Input: part model. Units: mm. Frame: model coordinates. Face numbers are marked on the shaded views. A direction names the side the tool comes from. Round coordinates to 2 decimals unless told otherwise and drop trailing zeros. Order: outer loops, then holes, each group sorted by start corner. A loop starts at its lowest first (then second) coordinate and runs counter-clockwise, first axis right, second up. Notation, with made-up numbers: (72.5, 29.5) - (103.5, 29.5) arc R18 ccw to (103.5, 37.5) - close; hole circle Ø11 at (87.25, 61.5). An arc over 180 degrees is marked (long way). One line per item, written item: value. Start each with the question number.
from build123d import *
from build123d.topology import SkipClean

# Parameters (mm, degrees)
BOSS_EXTRUDE1_DEPTH = 3.3
SKETCH2_R           = 8.19
BOSS_EXTRUDE2_DEPTH = 2.6
BOSS_EXTRUDE3_DEPTH = 1.2
BOSS_EXTRUDE4_DEPTH = 1
SKETCH7_R           = 5.575
BOSS_EXTRUDE5_DEPTH = 1
BOSS_EXTRUDE6_DEPTH = 1.6
BOSS_EXTRUDE7_DEPTH = 3.3
SKETCH9_R           = 3.43
BOSS_EXTRUDE8_DEPTH = 6.5
BOSS_EXTRUDE9_START = 0.65
BOSS_EXTRUDE9_DEPTH = 0.65


with BuildPart() as part:
    # Sketch1 → Boss-Extrude1 (new body)
    with BuildSketch(Plane(origin=(0, 0, 0), x_dir=(1, 0, 0), z_dir=(0, 1, 0))):
        with BuildLine():
            Line((8.141120253, -0.893454545), (6.690358093, -0.893454545))
            Line((6.690358093, -0.893454545), (6.690358093, 0.906545455))
            Line((6.690358093, 0.906545455), (8.139672926, 0.906545455))
            ThreePointArc((8.139672926, 0.906545455), (-8.189997352, -0.006585337), (8.141120253, -0.893454545))
        make_face()
    extrude(amount=BOSS_EXTRUDE1_DEPTH)

    # Sketch2 → Boss-Extrude2 (add)
    with BuildSketch(Plane(origin=(0, 3.3, 0), x_dir=(1, 0, 0), z_dir=(0, 1, 0))):
        with Locations(Location((0, 0, 0), (0, 0, 6.355052824))):
            Circle(SKETCH2_R)
    extrude(amount=BOSS_EXTRUDE2_DEPTH)

    # Sketch3 → Boss-Extrude3 (add)
    with BuildSketch(Plane(origin=(0, 5.9, 0), x_dir=(1, 0, 0), z_dir=(0, 1, 0))):
        with BuildLine():
            Line((7.8, 11.7), (-7.8, 11.7))
            Line((-7.8, 11.7), (-7.8, 3.501785259))
            ThreePointArc((-7.8, 3.501785259), (0, -8.55), (7.8, 3.501785259))
            Line((7.8, 3.501785259), (7.8, 11.7))
        make_face()
    extrude(amount=BOSS_EXTRUDE3_DEPTH)

    # Sketch4 → Boss-Extrude4 (add)
    with BuildSketch(Plane(origin=(0, 7.1, 0), x_dir=(1, 0, 0), z_dir=(0, 1, 0))):
        with BuildLine():
            Line((5.165208127, 5.575), (-5.165208127, 5.575))
            ThreePointArc((-5.165208127, 5.575), (-7.6, 0), (-5.165208127, -5.575))
            Line((-5.165208127, -5.575), (5.165208127, -5.575))
            ThreePointArc((5.165208127, -5.575), (7.6, 0), (5.165208127, 5.575))
        make_face()
    extrude(amount=BOSS_EXTRUDE4_DEPTH)

    # Sketch7 → Boss-Extrude5 (add)
    with BuildSketch(Plane(origin=(0, 8.1, 0), x_dir=(1, 0, 0), z_dir=(0, 1, 0))):
        with Locations(Location((0, 0, 0), (0, 0, 270))):
            Circle(SKETCH7_R)
    extrude(amount=BOSS_EXTRUDE5_DEPTH)

    # Sketch6 → Boss-Extrude6 (add)
    with SkipClean():  # the faces are left unmerged after this step: merging them gives an invalid solid
        with BuildSketch(Plane(origin=(0, 7.1, 0), x_dir=(1, 0, 0), z_dir=(0, 1, 0))):
            with BuildLine():
                Line((8.234834546, 2.3), (5.485974002, 0.992327692))
                ThreePointArc((5.485974002, 0.992327692), (5.575, 0), (5.485974002, -0.992327692))
                Line((5.485974002, -0.992327692), (8.234834546, -2.3))
                ThreePointArc((8.234834546, -2.3), (8.55, 0), (8.234834546, 2.3))
            make_face()
            with BuildLine():
                Line((-5.485974002, -0.992327692), (-8.234834546, -2.3))
                ThreePointArc((-8.234834546, -2.3), (-8.55, 0), (-8.234834546, 2.3))
                Line((-8.234834546, 2.3), (-5.485974002, 0.992327692))
                ThreePointArc((-5.485974002, 0.992327692), (-5.575, 0), (-5.485974002, -0.992327692))
            make_face()
        extrude(amount=BOSS_EXTRUDE6_DEPTH)

    # Sketch8 → Boss-Extrude7 (add)
    with SkipClean():  # the faces are left unmerged after this step: merging them gives an invalid solid
        with BuildSketch(Plane(origin=(0, 8.7, 0), x_dir=(1, 0, 0), z_dir=(0, 1, 0))):
            with BuildLine():
                Line((7.35, 0.79614814), (7.35, -0.79614814))
                ThreePointArc((7.35, -0.79614814), (7.807638503, -1.379024154), (8.482458308, -1.072763351))
                ThreePointArc((8.482458308, -1.072763351), (8.55002457, 0), (8.482458308, 1.072763351))
                ThreePointArc((8.482458308, 1.072763351), (7.807638503, 1.379024154), (7.35, 0.79614814))
            make_face()
        extrude(amount=BOSS_EXTRUDE7_DEPTH)

    # Sketch9 → Boss-Extrude8 (add)
    with SkipClean():  # the faces are left unmerged after this step: merging them gives an invalid solid
        with BuildSketch(Plane(origin=(0, 9.1, 0), x_dir=(1, 0, 0), z_dir=(0, 1, 0))):
            with Locations(Location((0, 0, 0), (0, 0, 90))):
                Circle(SKETCH9_R)
        extrude(amount=BOSS_EXTRUDE8_DEPTH)

    # Sketch13 → Boss-Extrude9 (add)
    with SkipClean():  # the faces are left unmerged after this step: merging them gives an invalid solid
        with BuildSketch(Plane.XZ.offset(-5.9).offset(BOSS_EXTRUDE9_START)):
            with BuildLine():
                Line((1.825, -7.98407634), (1.825, -12.95))
                Line((1.825, -12.95), (0.4975, -12.95))
                Line((0.4975, -12.95), (0.4975, -16.95))
                Line((0.4975, -16.95), (-0.5025, -16.95))
                Line((-0.5025, -16.95), (-0.5025, -12.95))
                Line((-0.5025, -12.95), (-1.83, -12.95))
                Line((-1.83, -12.95), (-1.83, -7.982931792))
                ThreePointArc((-1.83, -7.982931792), (-0.002564663, -8.189999598), (1.825, -7.98407634))
            make_face()
            with BuildLine():
                Line((4.884652449, -16.95), (4.884652449, -12.95))
                Line((4.884652449, -12.95), (3.557152449, -12.95))
                Line((3.557152449, -12.95), (3.557152449, -7.37717876))
                ThreePointArc((3.557152449, -7.37717876), (5.661322251, -5.9182371), (7.212152449, -3.880844889))
                Line((7.212152449, -3.880844889), (7.212152449, -12.95))
                Line((7.212152449, -12.95), (5.884652449, -12.95))
                Line((5.884652449, -12.95), (5.884652449, -16.95))
                Line((5.884652449, -16.95), (4.884652449, -16.95))
            make_face()
            with BuildLine():
                Line((-5.889652449, -16.95), (-4.889652449, -16.95))
                Line((-4.889652449, -16.95), (-4.889652449, -12.95))
                Line((-4.889652449, -12.95), (-3.562152449, -12.95))
                Line((-3.562152449, -12.95), (-3.562152449, -7.374765754))
                ThreePointArc((-3.562152449, -7.374765754), (-5.667142471, -5.912664054), (-7.217152449, -3.871538522))
                Line((-7.217152449, -3.871538522), (-7.217152449, -12.95))
                Line((-7.217152449, -12.95), (-5.889652449, -12.95))
                Line((-5.889652449, -12.95), (-5.889652449, -16.95))
            make_face()
        extrude(amount=-BOSS_EXTRUDE9_DEPTH)


solid = part.part
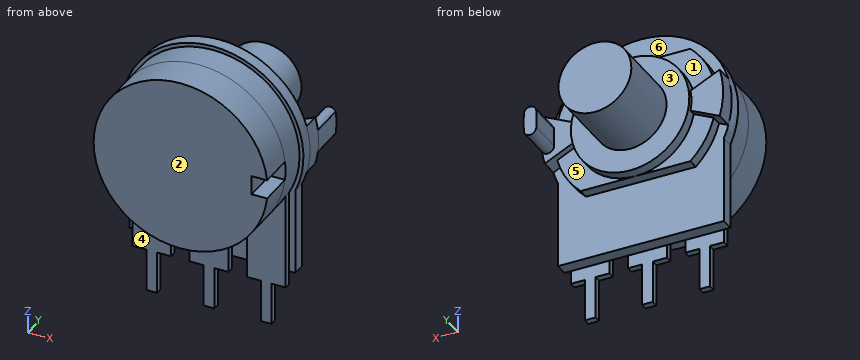
1. Line query: line 1 (Z direction, x = 1.75, y = 7.5) (3 decimals); line 2 (Y direction, x = -1, z = -8.75); line 3 (Y direction, x = 7.25, z = 0.5). Output: solid intervals per line, ascending. Write a range as from..to.
2. Section C-C (y = 13). Return the cut outline in (x, z).
3. Pull-direction query (X, two-part tool) for the marked faces 1 and 2; classes: released by +X, released by -X, zero draft, split by the parting line, or undercut.
4. Section D-D (x = -1.5). Return the cut outline in (y, z) (3 decimals).
5. Set-up query: the marked faces 3, 4, 5 and 6. Return all of +Z, -Z, +X, -X, +Y, -Y with unobstructed straight access to the full face (end or side cutting, diameter ignored); none if empty.
6. Section A-A (z = -12). Return the cut outline in (x, y) (3 decimals), then the cut area to 3 significant figures.
7. Pin query (flat end, axial travel): pin 1 (0.8 mm diameter, centred on x = 2, y = 8, fed in from -Z) (3 decimals); pin 2 (8 mm diameter, centred on y = 2, z = -5, fed in from -X); pin 3 (1.8 mm diameter, centred on x = -5.5, z = -14, fed in from +Y); pin 4 (4 mm diameter, centred on y = 13, z = -5.5, fed in from +X). Return the tip coordinate at first contact, or that it passes through.
Solved:
1. line 1: z = -5.575..5.575
1. line 2: y = 5.25..7.1
1. line 3: y = 3.3..8.7
2. outline: circle Ø6.86 at (0, 0)
3. face 1: undercut
3. face 2: zero draft
4. outline: (0, -8.051) - (5.25, -8.051) - (5.25, -12.95) - (5.9, -12.95) - (5.9, -11.7) - (7.1, -11.7) - (7.1, -5.575) - (8.1, -5.575) - (8.1, -5.369) - (9.1, -5.369) - (9.1, -3.085) - (15.6, -3.085) - (15.6, 3.085) - (9.1, 3.085) - (9.1, 5.369) - (8.1, 5.369) - (8.1, 5.575) - (7.1, 5.575) - (7.1, 8.417) - (5.9, 8.417) - (5.9, 8.051) - (0, 8.051) - close
5. face 3: +Y
5. face 4: -Z, -X, -Y
5. face 5: -Z, +Y
5. face 6: +Z, +Y
6. outline: (-7.217, 5.25) - (-3.562, 5.25) - (-3.562, 5.9) - (-7.217, 5.9) - close; (-1.83, 5.25) - (1.825, 5.25) - (1.825, 5.9) - (-1.83, 5.9) - close; (3.557, 5.25) - (7.212, 5.25) - (7.212, 5.9) - (3.557, 5.9) - close
6. area: 7.13 mm²
7. pin 1: stops at z = -5.575
7. pin 2: stops at x = -8.13
7. pin 3: stops at y = 5.9
7. pin 4: passes through
